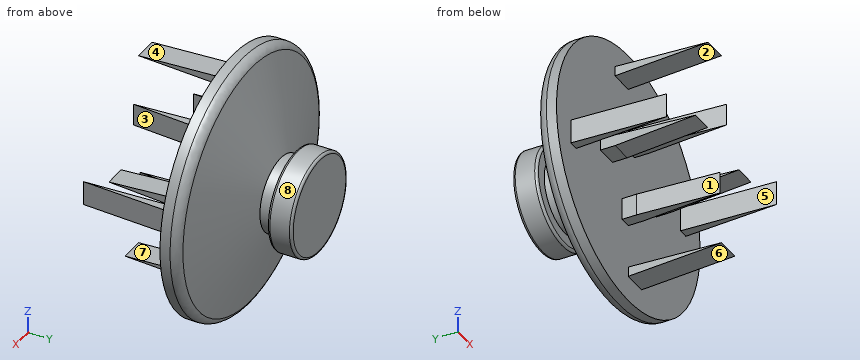
```python
from build123d import *

# Parameters (mm, degrees)
F0_R         = 67.2715048221
F1_DEPTH     = 25.4
F2_SIZE2     = 47.9485215904
F2_SIZE      = 16.51
F3_DEPTH     = 7.62
F4_R         = 25.9737658724
F5_DEPTH     = 12.7
F6_W         = 12.5492112711
F6_H         = 5.0823129714
F6_W_2       = 5.8439155109
F6_H_2       = 11.3746980205
F6_W_3       = 5.0823129714
F6_H_3       = 12.5492112711
F6_W_4       = 11.3746980205
F6_H_4       = 5.8439155109
F7_DEPTH     = 50.8
F8_T4_DEPTH  = 276.6958225406
F8_T9_DEPTH  = 276.6958225406
F9_T4_DEPTH  = 235.8904693574
F9_T9_DEPTH  = 235.8904693574
F10_T1_DEPTH = 123.632583689
F11_T4_DEPTH = 235.8904693574
F11_T9_DEPTH = 235.8904693574
F12_T4_DEPTH = 235.8904693574
F12_T9_DEPTH = 235.8904693574
F13_T4_DEPTH = 276.6958225406
F13_T9_DEPTH = 276.6958225406
F14_T4_DEPTH = 276.6958225406
F14_T9_DEPTH = 276.6958225406
F15_T4_DEPTH = 276.6958225406
F15_T9_DEPTH = 276.6958225406
F16_R        = 5.08
F17_R        = 1.27


# Not quite as in the source:
# - a fillet or chamfer that OpenCascade refuses, or shapes differently, is made with other operations: its cross-section is extruded or revolved along the edge and cut away or added


with BuildPart() as f1:
    # F0 (on Front) → F1 (new body)
    with BuildSketch(Plane.XZ):
        Circle(F0_R)
    extrude(amount=-F1_DEPTH)

    # F2
    f2_edges = [f1.edges().sort_by_distance(p)[0] for p in [
        (-67.271505, 25.4, 0),
    ]]
    f2_side = f1.faces().sort_by_distance((-67.271505, 12.7, 0))[0]
    chamfer(f2_edges, length=F2_SIZE, length2=F2_SIZE2, reference=f2_side)

    # F3 (add): a face of the model
    f3_faces = [f1.faces().sort_by_distance(p)[0] for p in [
        (0, 25.4, 0),
    ]]
    extrude(f3_faces, amount=F3_DEPTH)

    # F4 (on face) → F5 (join)
    with BuildSketch(Plane(origin=(0, 33.02, 0), x_dir=(-1, 0, 0), z_dir=(0, 1, 0))):
        Circle(F4_R)
    extrude(amount=F5_DEPTH)

    # F6 (on face) → F7 (join)
    with BuildSketch(Plane.XZ):
        with Locations((-6.2746056356, 51.3789299875)):
            Rectangle(F6_W, F6_H)
        with Locations((2.9219577555, 20.4010321759)):
            Rectangle(F6_W_2, F6_H_2)
        with Locations((-51.3789299875, -6.2746056356)):
            Rectangle(F6_W_3, F6_H_3)
        with Locations((-20.4010321759, 2.9219577555)):
            Rectangle(F6_W_4, F6_H_4)
        with Locations((6.2746056356, -51.3789299875)):
            Rectangle(F6_W, F6_H)
        with Locations((-2.9219577555, -20.4010321759)):
            Rectangle(F6_W_2, F6_H_2)
        with Locations((51.3789299875, 6.2746056356)):
            Rectangle(F6_W_3, F6_H_3)
        with Locations((20.4010321759, -2.9219577555)):
            Rectangle(F6_W_4, F6_H_4)
    extrude(amount=F7_DEPTH)

    # F8: chamfer of 50.8 x 2.6623151876 on 2 edges, made by hand


with BuildPart() as f8_tool2:
    # F8_s3 → F8_t4 (new body)
    with BuildSketch(Plane.YZ.offset(132.0733056347)):
        Polygon((0, 53.9200864732), (-50.8, 51.2577712856), (-50.8, 53.9200864732), align=None)
    extrude(amount=-F8_T4_DEPTH)

    split(bisect_by=Plane.XZ, keep=Keep.TOP)


with BuildPart() as f1_1:
    add(f1.part)

    # F8_t1: cut F8_tool2
    add(f8_tool2.part, mode=Mode.SUBTRACT)


with BuildPart() as f8_tool7:
    # F8_s8 → F8_t9 (new body)
    with BuildSketch(Plane.YZ.offset(-144.6225169058)):
        Polygon((0, 48.8377735019), (-50.8, 51.5000886895), (-50.8, 48.8377735019), align=None)
    extrude(amount=F8_T9_DEPTH)

    split(bisect_by=Plane.XZ, keep=Keep.TOP)


with BuildPart() as f1_2:
    add(f1_1.part)

    # F8_t6: cut F8_tool7
    add(f8_tool7.part, mode=Mode.SUBTRACT)

    # F9: chamfer of 43.18 x 3.0194397397 on 2 edges, made by hand


with BuildPart() as f9_tool2:
    # F9_s3 → F9_t4 (new body)
    with BuildSketch(Plane.XY.offset(-97.5442025028)):
        Polygon((2.8244757712, -50.8), (5.8439155109, -7.62), (5.8439155109, -50.8), align=None)
    extrude(amount=F9_T4_DEPTH)

    split(bisect_by=Plane.XY.offset(-48.8377735019), keep=Keep.TOP)


with BuildPart() as f1_3:
    add(f1_2.part)

    # F9_t1: cut F9_tool2
    add(f9_tool2.part, mode=Mode.SUBTRACT)


with BuildPart() as f9_tool7:
    # F9_s8 → F9_t9 (new body)
    with BuildSketch(Plane.XY.offset(138.3462668546)):
        Polygon((3.0194397397, -50.8), (0, -7.62), (0, -50.8), align=None)
    extrude(amount=-F9_T9_DEPTH)

    split(bisect_by=Plane.XY.offset(-26.0883811861), keep=Keep.TOP)


with BuildPart() as f1_4:
    add(f1_3.part)

    # F9_t6: cut F9_tool7
    add(f9_tool7.part, mode=Mode.SUBTRACT)

    # F10: chamfer of 43.18 x 3.0194397397 on 2 edges, made by hand

    # F10_s2 → F10_t1 (cut)
    with BuildSketch(Plane.YZ.offset(-138.3462668546)):
        Polygon((-7.62, 0), (-50.8, 3.0194397397), (-50.8, 0), align=None)
        Polygon((-50.8, 2.8244757712), (-7.62, 5.8439155109), (-50.8, 5.8439155109), align=None)
    extrude(amount=F10_T1_DEPTH, mode=Mode.SUBTRACT)

    # F11: chamfer of 43.18 x 3.0194397397 on 2 edges, made by hand


with BuildPart() as f11_tool2:
    # F11_s3 → F11_t4 (new body)
    with BuildSketch(Plane.XY.offset(97.5442025028)):
        Polygon((-2.8244757712, -50.8), (-5.8439155109, -7.62), (-5.8439155109, -50.8), align=None)
    extrude(amount=-F11_T4_DEPTH)

    split(bisect_by=Plane(origin=(0, 2.5524687068, 48.7040042853), x_dir=(1, 0, 0), z_dir=(0, -0.0523359562, -0.9986295348)), keep=Keep.TOP)


with BuildPart() as f1_5:
    add(f1_4.part)

    # F11_t1: cut F11_tool2
    add(f11_tool2.part, mode=Mode.SUBTRACT)


with BuildPart() as f11_tool7:
    # F11_s8 → F11_t9 (new body)
    with BuildSketch(Plane.XY.offset(-138.3462668546)):
        Polygon((0, -7.62), (-3.0194397397, -50.8), (0, -50.8), align=None)
    extrude(amount=F11_T9_DEPTH)

    split(bisect_by=Plane(origin=(0, 2.5524687068, 48.7040042853), x_dir=(1, 0, 0), z_dir=(0, -0.0523359562, -0.9986295348)), keep=Keep.TOP)


with BuildPart() as f1_6:
    add(f1_5.part)

    # F11_t6: cut F11_tool7
    add(f11_tool7.part, mode=Mode.SUBTRACT)

    # F12: chamfer of 43.18 x 3.0194397397 on 2 edges, made by hand


with BuildPart() as f12_tool2:
    # F12_s3 → F12_t4 (new body)
    with BuildSketch(Plane.YZ.offset(-97.5442025028)):
        Polygon((-50.8, -2.8244757712), (-7.62, -5.8439155109), (-50.8, -5.8439155109), align=None)
    extrude(amount=F12_T4_DEPTH)

    split(bisect_by=Plane.YZ.offset(-48.8377735019), keep=Keep.TOP)


with BuildPart() as f1_7:
    add(f1_6.part)

    # F12_t1: cut F12_tool2
    add(f12_tool2.part, mode=Mode.SUBTRACT)


with BuildPart() as f12_tool7:
    # F12_s8 → F12_t9 (new body)
    with BuildSketch(Plane.YZ.offset(138.3462668546)):
        Polygon((-7.62, 0), (-50.8, -3.0194397397), (-50.8, 0), align=None)
    extrude(amount=-F12_T9_DEPTH)

    split(bisect_by=Plane.YZ.offset(-48.8377735019), keep=Keep.TOP)


with BuildPart() as f1_8:
    add(f1_7.part)

    # F12_t6: cut F12_tool7
    add(f12_tool7.part, mode=Mode.SUBTRACT)

    # F13: chamfer of 50.8 x 2.6623151876 on 2 edges, made by hand


with BuildPart() as f13_tool2:
    # F13_s3 → F13_t4 (new body)
    with BuildSketch(Plane.XY.offset(132.0733056347)):
        Polygon((-51.5000886895, -50.8), (-48.8377735019, 0), (-48.8377735019, -50.8), align=None)
    extrude(amount=-F13_T4_DEPTH)

    split(bisect_by=Plane.XZ, keep=Keep.TOP)


with BuildPart() as f1_9:
    add(f1_8.part)

    # F13_t1: cut F13_tool2
    add(f13_tool2.part, mode=Mode.SUBTRACT)


with BuildPart() as f13_tool7:
    # F13_s8 → F13_t9 (new body)
    with BuildSketch(Plane.XY.offset(132.0733056347)):
        Polygon((-51.2577712856, -50.8), (-53.9200864732, 0), (-53.9200864732, -50.8), align=None)
    extrude(amount=-F13_T9_DEPTH)

    split(bisect_by=Plane.XZ, keep=Keep.TOP)


with BuildPart() as f1_10:
    add(f1_9.part)

    # F13_t6: cut F13_tool7
    add(f13_tool7.part, mode=Mode.SUBTRACT)

    # F14: chamfer of 50.8 x 2.6623151876 on 2 edges, made by hand


with BuildPart() as f14_tool2:
    # F14_s3 → F14_t4 (new body)
    with BuildSketch(Plane.YZ.offset(-132.0733056347)):
        Polygon((-50.8, -51.2577712856), (0, -53.9200864732), (-50.8, -53.9200864732), align=None)
    extrude(amount=F14_T4_DEPTH)

    split(bisect_by=Plane.XZ, keep=Keep.TOP)


with BuildPart() as f1_11:
    add(f1_10.part)

    # F14_t1: cut F14_tool2
    add(f14_tool2.part, mode=Mode.SUBTRACT)


with BuildPart() as f14_tool7:
    # F14_s8 → F14_t9 (new body)
    with BuildSketch(Plane.YZ.offset(-132.0733056347)):
        Polygon((-50.8, -51.5000886895), (0, -48.8377735019), (-50.8, -48.8377735019), align=None)
    extrude(amount=F14_T9_DEPTH)

    split(bisect_by=Plane.XZ, keep=Keep.TOP)


with BuildPart() as f1_12:
    add(f1_11.part)

    # F14_t6: cut F14_tool7
    add(f14_tool7.part, mode=Mode.SUBTRACT)

    # F15: chamfer of 50.8 x 2.6623151876 on 2 edges, made by hand


with BuildPart() as f15_tool2:
    # F15_s3 → F15_t4 (new body)
    with BuildSketch(Plane.XY.offset(-132.0733056347)):
        Polygon((51.2577712856, -50.8), (53.9200864732, 0), (53.9200864732, -50.8), align=None)
    extrude(amount=F15_T4_DEPTH)

    split(bisect_by=Plane.XZ, keep=Keep.TOP)


with BuildPart() as f1_13:
    add(f1_12.part)

    # F15_t1: cut F15_tool2
    add(f15_tool2.part, mode=Mode.SUBTRACT)


with BuildPart() as f15_tool7:
    # F15_s8 → F15_t9 (new body)
    with BuildSketch(Plane.XY.offset(144.6225169058)):
        Polygon((48.8377735019, 0), (51.5000886895, -50.8), (48.8377735019, -50.8), align=None)
    extrude(amount=-F15_T9_DEPTH)

    split(bisect_by=Plane.XZ, keep=Keep.TOP)


with BuildPart() as f1_14:
    add(f1_13.part)

    # F15_t6: cut F15_tool7
    add(f15_tool7.part, mode=Mode.SUBTRACT)

    # F16
    f16_edges = [f1_14.edges().sort_by_distance(p)[0] for p in [
        (-67.271505, 8.89, 0),
    ]]
    fillet(f16_edges, radius=F16_R)

    # F17
    f17_edges = [f1_14.edges().sort_by_distance(p)[0] for p in [
        (25.973766, 45.72, 0),
        (25.973766, 33.02, 0),
    ]]
    fillet(f17_edges, radius=F17_R)


solid = f1_14.part
```
The model under review builds one solid part; all positions refer to its coordinate system, in mm. Face numbers are marked on the shaded views. A direction names the side the tool comes from. Give positions to 0.01 mm unless a question says otherwise; leave off trailing zeros. Write each loop counter-clockwise with the first axis right and the second up, starting at its lowest first coordinate (ties: lowest second). Pieces come first, ordered by that corner, then holes. Notation, with made-up numbers: (54.25, -34.75) -> (67.25, -34.75) arc R21 cw to (67.25, -28.75) -> close; hole circle Ø3 at (72.25, 10.5). An arc over 180 degrees is marked (long way). Put each result on its own line as item: value.
(1) We need section A-A, the plane y = -37. State how many separate pieces and enclosed holes the cut face has, and give its area (3 significant figures).
Results are:
separate pieces: 8
enclosed holes: 0
area: 139 mm²
(2) For pin 1 Ø1.5 at (x, y) = (51, -13) entering from -Z; pin 2 Ø5.5 at (x, y) = (50.5, -24.5) entering from +Z; pin 3 Ø10 at (x, z) = (-40, 52.5) entering from +Y, all flat-tipped, find the tip position at first contact; note any pin that passes through.
Results are:
pin 1: z = 0
pin 2: z = 12.55
pin 3: y = 11.05
(3) The part is to be moulded in two halves that separate along Z. For the marked faces 5, 6, 7 and 8, say which applies: pulls with the +Z half, pulls with the -Z half, needs draft (parallel to the pull), parting line crosses it, or undercut.
Results are:
face 5: needs draft
face 6: pulls with the -Z half
face 7: undercut
face 8: parting line crosses it
(4) To check wall thickness, follow probe 1 along Z at (x, y) = (-8, 42); probe 2 along Z at (x, y) = (-23.5, -5); probe 3 along Y at (x, z) = (-10, 17.5). State the ranges of each line that lie inside material, in increasing order. Write a range as from..to.
Results are:
probe 1: -24.71..24.71
probe 2: 0..5.84
probe 3: 0..25.11, 33.02..45.72
(5) Tool access review of the marked faces 1, 2, 3 and 4: name each direction out of +Z, -Z, +X, -X, +Y, -Y from which nothing blocks a thin tool from reaching the whole face with its end or side.
Results are:
face 1: -Z, -X, -Y
face 2: +X, -X, -Y
face 3: +Z, +X, -Y
face 4: +Z, +X, -X, -Y
(6) We need section B-B, the plane y = 19.5. Give the boundary of the cut face in (x, z), and give its area (3 significant figures).
Results are:
outline: circle Ø72.92 at (0, 0)
area: 4,180 mm²
